```python
from build123d import *

# Parameters (mm, degrees)
BOSS_EXTRUDE1_DEPTH = 12.7
CUT_EXTRUDE1_REACH  = 14.7
SKETCH2_R           = 0.775
SKETCH4_R           = 12.5
SKETCH4_R_2         = 2.6
BOSS_EXTRUDE3_DEPTH = 20.5


with BuildPart() as part:
    # Sketch1 → Boss-Extrude1 (new body)
    with BuildSketch(Plane(origin=(0, 0, 0), x_dir=(-1, 0, 0), z_dir=(0, 0, -1))):
        Polygon((22.52557458, -1.736588639), (22.52557458, 0.194536921), (19.229808022, 0.93665661), (15.128723263, 11.851737372), (17.063649078, 14.621011813), (15.786423571, 16.069438867), (12.890863827, 14.329165151), (2.313040546, 19.235032954), (1.719665356, 22.560799741), (-0.211460204, 22.560799741), (-0.98374926, 19.271971918), (-11.902473648, 15.180597821), (-14.673902719, 17.112436257), (-16.073066924, 15.781427071), (-14.308800518, 12.900423272), (-19.236913758, 2.332945609), (-22.560976284, 1.730096406), (-22.560976284, -0.201029153), (-19.275488766, -0.987407309), (-15.174404006, -11.902488071), (-17.112216048, -14.669743631), (-15.788139908, -16.075470597), (-12.910837913, -14.305173427), (-2.333014633, -19.21104123), (-1.727718406, -22.534659035), (0.203407153, -22.534659035), (0.978499423, -19.246490729), (11.89722381, -15.155116632), (14.659649692, -17.099807376), (16.072878525, -15.783741196), (14.276312796, -12.922767512), (19.204426036, -2.355289849), align=None)
    extrude(amount=-BOSS_EXTRUDE1_DEPTH)

    # Sketch2 → Cut-Extrude1 (cut, up to next)
    with BuildSketch(Plane(origin=(0, 0, 0), x_dir=(-1, 0, 0), z_dir=(0, 0, -1)), mode=Mode.PRIVATE) as cut_extrude1_sk1:
        with Locations((-0.019773646, -0.00956531)):
            Circle(SKETCH2_R)
    cut_extrude1_tool1 = extrude(cut_extrude1_sk1.sketch, amount=-CUT_EXTRUDE1_REACH, mode=Mode.PRIVATE) & part.part
    add(cut_extrude1_tool1.solids().sort_by_distance((0.019774, -0.009565, 0))[0], mode=Mode.SUBTRACT)

    # Sketch4 → Boss-Extrude3 (add)
    with BuildSketch(Plane(origin=(0, 0, 0), x_dir=(-1, 0, 0), z_dir=(0, 0, -1))):
        Circle(SKETCH4_R)
        Circle(SKETCH4_R_2, mode=Mode.SUBTRACT)
    extrude(amount=BOSS_EXTRUDE3_DEPTH)


solid = part.part
```
Build history of the part. All positions in model axes, mm. A direction names the side the tool comes from. Round coordinates to 2 decimals unless told otherwise and drop trailing zeros. Write each loop counter-clockwise with the first axis right and the second up, starting at its lowest first coordinate (ties: lowest second). Pieces come first, ordered by that corner, then holes. Notation, with made-up numbers: (44, -35) - (63, -35) arc R19 cw to (63, -4) - close; hole circle Ø7 at (60.5, 88). An arc over 180 degrees is marked (long way). Write each question's results on one line, items separated by ' | '. Start each with the question number.
Item 1: Mould opens along Y. For faces 1 (the face through (0.635, -0.481, 6.261)), 2 (the face through (-22.526, -1, 6)), 3 (the face through (-6.36, -17.23, 6.26)), 4 (the face through (-17.208, 6.318, 6.261)) say: pulls with the +Y half, pulls with the -Y half, needs draft (parallel to the pull), parting line crosses it, or undercut.
Item 2: Saw through at B-B (y = 7). Write the cut outline in (x, z), and give its area (3 significant figures).
Item 3: Wall check: L1, parallel to X at y = 0, z = 7; L2, parallel to Y at x = 0, z = -6; L3, parallel to Z at x = 8, y = 15. Give the ranges that are in metal, low to high. Write a range as [from, to].
Item 4: Which spindle directions (+Z, -Z, +X, -X, +Y, -Y) get a long thin tool onto all of the face, cutting with end or side? Do faces 5 (the face through (6.367, 17.255, 6.261)), 6 (the face through (-10, 10, 0)), 7 (the face through (14.37, -15.203, 6.261)), 8 (the face through (15.36, 16.46, 6.26)), 9 (the face through (-16.083, 13.217, 6.261)). Say none if no direction does.
Item 5: Saw through at C-C (x = 6). Write the cut outline in (y, z), and give its area (3 significant figures).
Item 6: Drop flat-ended pins along their axis: P1, Ø1.5, axis at x = 7.5, z = -14.5, coming from the -Y side; P2, Ø1.6, axis at x = -1, y = 1, coming from the -Z side; P3, Ø1.5, axis at x = -0.5, z = -3.5, coming from the -Y side; P4, Ø2, axis at y = 15, z = -6, coming from the -X side. Give the stop position or say it passes through.
Item 7: Saw through at D-D (z = -18). Write the cut outline in (x, y), and give its area (3 significant figures).
Results are:
1) face 1: undercut | face 2: needs draft | face 3: pulls with the -Y half | face 4: undercut
2) outline: (-16.95, 0) - (-10.36, 0) - (-10.36, -20.5) - (10.36, -20.5) - (10.36, 0) - (17.06, 0) - (17.06, 12.7) - (-16.95, 12.7) - close | area: 857 mm²
3) L1: x = [-22.53, -0.76], [0.79, 22.56] | L2: y = [-12.5, -2.6], [2.6, 12.5] | L3: z = [0, 12.7]
4) face 5: +Z, -Z, +Y | face 6: -Z | face 7: +Z, -Z, -Y | face 8: +Z, -Z, +X, +Y | face 9: +Z, -Z, -X
5) outline: (-17.51, 0) - (-10.97, 0) - (-10.97, -20.5) - (10.97, -20.5) - (10.97, 0) - (17.39, 0) - (17.39, 12.7) - (-17.51, 12.7) - close | area: 893 mm²
6) P1: stops at y = -10.52 | P2: stops at z = 0 | P3: stops at y = -12.5 | P4: passes through
7) outline: circle Ø25 at (0, 0); hole circle Ø5.2 at (0, 0) | area: 470 mm²
